Build history of the part. All positions in model axes, mm. Face numbers are marked on the shaded views. A direction names the side the tool comes from. Give positions to 0.01 mm unless a question says otherwise; leave off trailing zeros. Write each loop counter-clockwise with the first axis right and the second up, starting at its lowest first coordinate (ties: lowest second). Pieces come first, ordered by that corner, then holes. Notation, with made-up numbers: (-20, -31.75) -> (32, -31.75) arc R21 ccw to (32, -23.75) -> close; hole circle Ø1 at (45, 49). An arc over 180 degrees is marked (long way). One line per question, with ' | ' between items. Start each with the question number.
(1) Band-saw the part on C-C, the plane x = 0. Give the cut face in (y, z), and give its area (3 significant figures).
(2) Band-saw the part on B-B, the plane y = -2.75. Give the cut face in (x, z).
(3) Band-saw the part on D-D, the plane y = -1. Give the cut face in (x, z).
(4) Band-saw the part on A-A, the plane z = 0. Give the cut face in (x, y).
(5) Tool access for the marked faces 1 and 2: list every direction of +Z, -Z, +X, -X, +Y, -Y with a clear straight run to the whole face (end or side of a thin tool).
(6) Drill centre lines: probe 1 along Y at (x, z) = (-0.75, 1); probe 2 along Y at (x, z) = (-3.5, 2.25); probe 3 along X at (y, z) = (2, -2.5). Where is each one in solid material? Low to high. Write a range as from..to.
(7) Pin check, flat tips, straight feed: P1, Ø2, axis at y = -1.5, z = -2.5, coming from the +X side; P2, Ø4.5, axis at x = 2.5, z = 2, coming from the +Y side; P3, Ø3, axis at y = 3.5, z = 1, coming from the -X side; P4, Ø5, axis at y = -3, z = 0, coming from the +X side. Stop position of each tip, or through.
from build123d import *

# Parameters (mm, degrees)
EXTRUDE_1_DEPTH = 0.7
SKETCH_2_R      = 4
EXTRUDE_2_DEPTH = 4.6
FILLET_1_R      = 1
SKETCH_4_R      = 0.2
EXTRUDE_3_DEPTH = 4.3
SKETCH_5_R      = 0.25
EXTRUDE_4_DEPTH = 2


with BuildPart() as part:
    # Эскиз1 → Бобышка-Вытянуть1 (new body)
    with BuildSketch(Plane(origin=(0, 0, 0), x_dir=(1, 0, 0), z_dir=(0, 1, 0))):
        with BuildLine():
            Line((0, -5.806112013), (0.5, -5.806112013))
            Line((0.5, -5.806112013), (0.5, -4.673328578))
            ThreePointArc((0.5, -4.673328578), (0, 4.7), (-0.5, -4.673328578))
            Line((-0.5, -4.673328578), (-0.5, -5.806112013))
            Line((-0.5, -5.806112013), (0, -5.806112013))
        make_face()
    extrude(amount=EXTRUDE_1_DEPTH)

    # Эскиз2 → Бобышка-Вытянуть2 (add)
    with BuildSketch(Plane(origin=(0, 0.7, 0), x_dir=(1, 0, 0), z_dir=(0, 1, 0))):
        with Locations(Location((0, 0, 0), (0, 0, 270))):
            Circle(SKETCH_2_R)
    extrude(amount=EXTRUDE_2_DEPTH)

    # Скругление1
    fillet_1_edges = [part.edges().sort_by_distance(p)[0] for p in [
        (0, 5.3, -4),
    ]]
    fillet(fillet_1_edges, radius=FILLET_1_R)

    # Эскиз4 → Бобышка-Вытянуть3 (add)
    with BuildSketch(Plane.XZ):
        with Locations(Location((2.5, 0, 0), (0, 0, 90))):
            Circle(SKETCH_4_R)
        with Locations(Location((1.767766953, -1.767766953, 0), (0, 0, 90))):
            Circle(SKETCH_4_R)
        with Locations(Location((0, -2.5, 0), (0, 0, 90))):
            Circle(SKETCH_4_R)
        with Locations(Location((-1.767766953, -1.767766953, 0), (0, 0, 90))):
            Circle(SKETCH_4_R)
        with Locations(Location((-2.5, 0, 0), (0, 0, 90))):
            Circle(SKETCH_4_R)
        with Locations(Location((-1.767766953, 1.767766953, 0), (0, 0, 90))):
            Circle(SKETCH_4_R)
        with Locations(Location((0, 2.5, 0), (0, 0, 90))):
            Circle(SKETCH_4_R)
        with Locations(Location((1.767766953, 1.767766953, 0), (0, 0, 90))):
            Circle(SKETCH_4_R)
    extrude(amount=EXTRUDE_3_DEPTH)

    # Эскиз5 → Бобышка-Вытянуть4 (add)
    with BuildSketch(Plane.XZ):
        with Locations(Location((0, 2.5, 0), (0, 0, 90))):
            Circle(SKETCH_5_R)
    extrude(amount=EXTRUDE_4_DEPTH)


solid = part.part
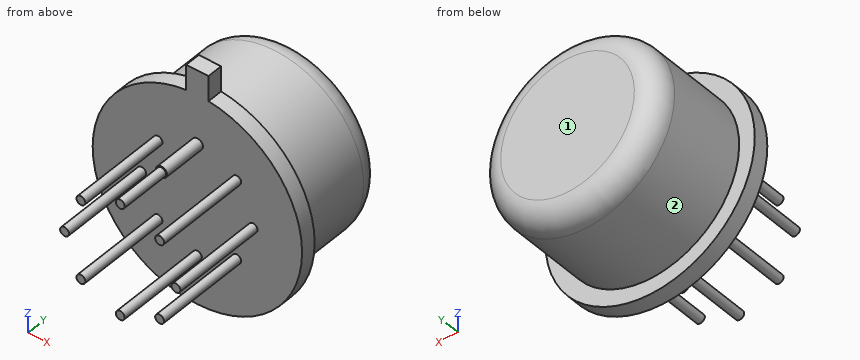
Results:
1) outline: (-4.3, -2.7) -> (0, -2.7) -> (0, -4.7) -> (0.7, -4.7) -> (0.7, -4) -> (4.3, -4) arc R1 ccw to (5.3, -3) -> (5.3, 3) arc R1 ccw to (4.3, 4) -> (0.7, 4) -> (0.7, 5.81) -> (0, 5.81) -> (0, 2.75) -> (-2, 2.75) -> (-2, 2.7) -> (-4.3, 2.7) -> (-4.3, 2.3) -> (-2, 2.3) -> (-2, 2.25) -> (0, 2.25) -> (0, -2.3) -> (-4.3, -2.3) -> close | area: 47.4 mm²
2) outline: circle Ø0.4 at (-2.5, 0); circle Ø0.4 at (-1.77, -1.77); circle Ø0.4 at (-1.77, 1.77); circle Ø0.4 at (0, -2.5); circle Ø0.4 at (0, 2.5); circle Ø0.4 at (1.77, -1.77); circle Ø0.4 at (1.77, 1.77); circle Ø0.4 at (2.5, 0)
3) outline: circle Ø0.4 at (-2.5, 0); circle Ø0.4 at (-1.77, -1.77); circle Ø0.4 at (-1.77, 1.77); circle Ø0.5 at (0, 2.5); circle Ø0.4 at (0, -2.5); circle Ø0.4 at (1.77, -1.77); circle Ø0.4 at (1.77, 1.77); circle Ø0.4 at (2.5, 0)
4) outline: (-4.7, 0) -> (-2.7, 0) -> (-2.7, -4.3) -> (-2.3, -4.3) -> (-2.3, 0) -> (2.3, 0) -> (2.3, -4.3) -> (2.7, -4.3) -> (2.7, 0) -> (4.7, 0) -> (4.7, 0.7) -> (4, 0.7) -> (4, 4.3) arc R1 ccw to (3, 5.3) -> (-3, 5.3) arc R1 ccw to (-4, 4.3) -> (-4, 0.7) -> (-4.7, 0.7) -> close
5) face 1: +Z, -Z, +X, -X, +Y | face 2: +Y
6) probe 1: y = 0..5.3 | probe 2: y = 0..0.7 | probe 3: x = -3.12..3.12
7) P1: stops at x = 1.97 | P2: stops at y = 5.3 | P3: stops at x = -4 | P4: stops at x = 2.7
